Here's how the part is built. I have some questions about the finished solid (model axes, mm). Face numbers are marked on the shaded views. A direction names the side the tool comes from. Give positions to 0.01 mm unless a question says otherwise; leave off trailing zeros. Loops run counter-clockwise (first coordinate to the right, second up) from the corner with the lowest first, then second, coordinate; pieces in that order, holes last. Notation, with made-up numbers: (-8, 89.25) - (27, 89.25) arc R35 ccw to (27, 126.25) - close; hole circle Ø5 at (19, 24). An arc over 180 degrees is marked (long way). Use a Markdown table: item, result.
from build123d import *

# Parameters (mm, degrees)
SKETCH1_W           = 12.5
SKETCH1_H           = 127
BOSS_EXTRUDE1_DEPTH = 106
SKETCH2_W           = 12.5
SKETCH2_H           = 35.5
CUT_EXTRUDE1_DEPTH  = 200
FILLET3_R           = 8
FILLET4_R           = 10
FILLET5_R           = 40
SKETCH5_R           = 3.5
CUT_EXTRUDE5_DEPTH  = 25
CUT_EXTRUDE6_START  = -6
SKETCH5_3_R         = 9.5
SKETCH5_3_R_2       = 3.5
CUT_EXTRUDE6_DEPTH  = 7
SKETCH4_R           = 1.55
CUT_EXTRUDE7_DEPTH  = 16


with BuildPart() as part:
    # Sketch1 → Boss-Extrude1 (new body)
    with BuildSketch(Plane.XY):
        Polygon((0, 8), (0, 0), (228, 0), (228, 8), (178.113248654, 8), (178.113248654, 7), (181, 2), (161, 2), (163.886751346, 7), (163.886751346, 8), (64.113248654, 8), (64.113248654, 7), (67, 2), (47, 2), (49.886751346, 7), (49.886751346, 8), align=None)
        with Locations((234.25, 63.5)):
            Rectangle(SKETCH1_W, SKETCH1_H)
        with Locations((-6.25, 63.5)):
            Rectangle(SKETCH1_W, SKETCH1_H)
    extrude(amount=-BOSS_EXTRUDE1_DEPTH)

    # Sketch2 → Cut-Extrude1 (cut)
    with BuildSketch(Plane(origin=(0, 127, 0), x_dir=(1, 0, 0), z_dir=(0, 1, 0))):
        with Locations((-6.25, 88.25)):
            Rectangle(SKETCH2_W, SKETCH2_H)
        with Locations((-6.25, 17.75)):
            Rectangle(SKETCH2_W, SKETCH2_H)
        with Locations((234.25, 88.25)):
            Rectangle(SKETCH2_W, SKETCH2_H)
        with Locations((234.25, 17.75)):
            Rectangle(SKETCH2_W, SKETCH2_H)
        with BuildLine():
            Line((109.95, 20), (109.95, 86))
            ThreePointArc((109.95, 86), (114, 90.05), (118.05, 86))
            Line((118.05, 86), (118.05, 20))
            ThreePointArc((118.05, 20), (114, 15.95), (109.95, 20))
        make_face()
    extrude(amount=-CUT_EXTRUDE1_DEPTH, mode=Mode.SUBTRACT)

    # Fillet3
    fillet3_edges = [part.edges().sort_by_distance(p)[0] for p in [
        (-6.25, 127, -35.5),
        (234.25, 127, -70.5),
        (234.25, 127, -35.5),
        (-6.25, 127, -70.5),
    ]]
    fillet(fillet3_edges, radius=FILLET3_R)

    # Fillet4
    fillet4_edges = [part.edges().sort_by_distance(p)[0] for p in [
        (228, 8, -53),
        (240.5, 0, -53),
        (0, 8, -53),
        (-12.5, 0, -53),
    ]]
    fillet(fillet4_edges, radius=FILLET4_R)

    # Fillet5
    # the kernel refuses this fillet: 40 mm, written as the material it takes off along each edge
    with BuildSketch(Plane(origin=(228, 107.36517247, -106), x_dir=(-1, 0, 0), z_dir=(0, -1, 0))) as fillet5_piece_1:
        with BuildLine():
            CenterArc((39.746068988, -40), FILLET5_R, 90, 83.540550223)
            Line((0, -35.5), (-0.79492138, -35.41))
            ThreePointArc((-0.79492138, -35.41), (-0.8, -17.75), (-0.8, 0))
            Line((-0.8, 0), (0, 0.8))
            Line((0, 0.8), (39.746068988, 0.8))
            Line((39.746068988, 0.8), (39.746068988, 0))
        make_face()
    extrude(amount=206.73034494, mode=Mode.SUBTRACT)
    with BuildSketch(Plane(origin=(0, 107.36517247, -106), x_dir=(0, 0, 1), z_dir=(0, -1, 0))) as fillet5_piece_2:
        with BuildLine():
            CenterArc((40, -39.746068988), FILLET5_R, 96.459449777, 83.540550223)
            Line((0, -39.746068988), (-0.8, -39.746068988))
            Line((-0.8, -39.746068988), (-0.8, 0))
            Line((-0.8, 0), (0, 0.8))
            ThreePointArc((0, 0.8), (17.75, 0.8), (35.41, 0.79492138))
            Line((35.41, 0.79492138), (35.5, 0))
        make_face()
    extrude(amount=206.73034494, mode=Mode.SUBTRACT)
    with BuildSketch(Plane(origin=(0, 107.36517247, 0), x_dir=(0, 0, -1), z_dir=(0, -1, 0))) as fillet5_piece_3:
        with BuildLine():
            CenterArc((40, 39.746068988), FILLET5_R, 180, 83.540550223)
            Line((0, 39.746068988), (-0.8, 39.746068988))
            Line((-0.8, 39.746068988), (-0.8, 0))
            Line((-0.8, 0), (0, -0.8))
            ThreePointArc((0, -0.8), (17.75, -0.8), (35.41, -0.79492138))
            Line((35.41, -0.79492138), (35.5, 0))
        make_face()
    extrude(amount=206.73034494, mode=Mode.SUBTRACT)
    with BuildSketch(Plane(origin=(228, 107.36517247, 0), x_dir=(-1, 0, 0), z_dir=(0, -1, 0))) as fillet5_piece_4:
        with BuildLine():
            CenterArc((39.746068988, 40), FILLET5_R, 186.459449777, 83.540550223)
            Line((0, 35.5), (-0.79492138, 35.41))
            ThreePointArc((-0.79492138, 35.41), (-0.8, 17.75), (-0.8, 0))
            Line((-0.8, 0), (0, -0.8))
            Line((0, -0.8), (39.746068988, -0.8))
            Line((39.746068988, -0.8), (39.746068988, 0))
        make_face()
    extrude(amount=206.73034494, mode=Mode.SUBTRACT)

    # Sketch5 → Cut-Extrude5 (cut)
    with BuildSketch(Plane(origin=(0, 0, 0), x_dir=(0, 0, -1), z_dir=(1, 0, 0))):
        with Locations((53, 108.5)):
            Circle(SKETCH5_R)
    extrude(amount=-CUT_EXTRUDE5_DEPTH, mode=Mode.SUBTRACT)

    # Sketch5<3> → Cut-Extrude6 (cut)
    with BuildSketch(Plane(origin=(0, 0, 0), x_dir=(0, 0, -1), z_dir=(1, 0, 0)).offset(CUT_EXTRUDE6_START)):
        with Locations((53, 108.5)):
            Circle(SKETCH5_3_R)
        with Locations((53, 108.5)):
            Circle(SKETCH5_3_R_2, mode=Mode.SUBTRACT)
    extrude(amount=-CUT_EXTRUDE6_DEPTH, mode=Mode.SUBTRACT)

    # Sketch4 → Cut-Extrude7 (cut)
    with BuildSketch(Plane(origin=(240.5, 0, 0), x_dir=(0, 0, -1), z_dir=(1, 0, 0))):
        with Locations((40.625, 120.875)):
            Circle(SKETCH4_R)
        with Locations((40.625, 96.125)):
            Circle(SKETCH4_R)
        with Locations((65.375, 96.125)):
            Circle(SKETCH4_R)
        with Locations((65.375, 120.875)):
            Circle(SKETCH4_R)
    extrude(amount=-CUT_EXTRUDE7_DEPTH, mode=Mode.SUBTRACT)


solid = part.part
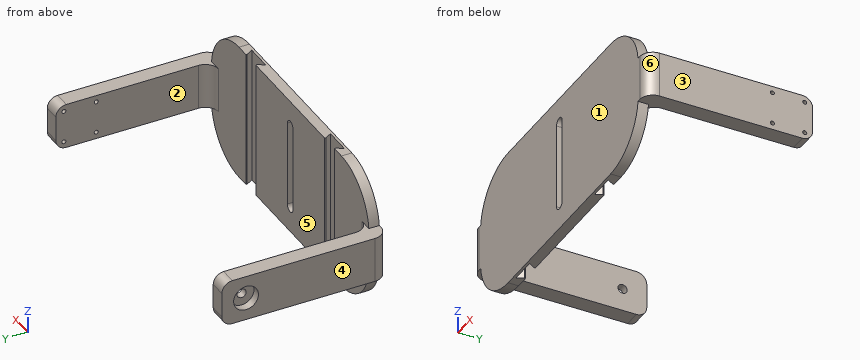
(1) We'd pull the mould along X, two halves only. Please class the marked faces 1, 2, 3 and 4: pulls with the +X half, pulls with the -X half, needs draft (parallel to the pull), parting line crosses it, or undercut.
A:
| item | result |
|---|---|
| face 1 | needs draft |
| face 2 | undercut |
| face 3 | pulls with the +X half |
| face 4 | pulls with the -X half |
(2) Suppose I cut it at B-B on y = 108.5. Write out the boundary of the cut face in (x, z), plus the area to 4 significant figures.
A:
| item | result |
|---|---|
| outline | (-12.5, -70.5) - (0, -70.5) - (0, -56.5) - (-6, -56.5) - (-6, -62.5) - (-12.5, -62.5) - close; (-12.5, -43.5) - (-6, -43.5) - (-6, -49.5) - (0, -49.5) - (0, -35.5) - (-12.5, -35.5) - close; (228, -70.5) - (240.5, -70.5) - (240.5, -35.5) - (228, -35.5) - close |
| area | 709.5 mm2 |
(3) Suppose I cut it at A-A on x = 114. Write out the boundary of the cut face in (y, z).
A:
| item | result |
|---|---|
| outline | (0, -106) - (8, -106) - (8, -90.05) - (0, -90.05) - close; (0, -15.95) - (8, -15.95) - (8, 0) - (0, 0) - close |
(4) Suppose I cut it at C-C on y = 47. Write out the boundary of the cut face in (x, z), plus the area to 3 significant figures.
A:
| item | result |
|---|---|
| outline | (-12.5, -70.5) - (0, -70.5) - (0, -35.5) - (-12.5, -35.5) - close; (228, -70.5) - (240.5, -70.5) - (240.5, -35.5) - (228, -35.5) - close |
| area | 875 mm2 |
(5) Will these pins go through, and if not, where does the flat tip stop? pin 1 (22 mm diameter, centred on x = 52.5, z = -59, fed in from +Y); pin 2 (25 mm diameter, centred on x = 224.5, y = 75.5, fed in from +Z); pin 3 (5.5 mm diameter, centred on y = 108.5, z = -53, fed in from -X).
A:
| item | result |
|---|---|
| pin 1 | y = 8 |
| pin 2 | z = -35.5 |
| pin 3 | x = 228 |
(6) On a 3-axis mill with a long thin cutter (end or side, diameter ignored), from which of +Z, -Z, +X, -X, +Y, -Y can I reach the whole of each face in a straight line? I mean the marked faces 5 and 6. Say none if no direction works.
A:
| item | result |
|---|---|
| face 5 | +Z, -Z, +Y |
| face 6 | +Z, -Z, +X, -Y |
(7) If I drill on line 1 (X direction, y = 111, z = -50); line 2 (X direction, y = 101, z = -46); line 3 (Y direction, x = 141, z = -54.5), over which ranges is the centre line in solid material (lowest first)?
A:
| item | result |
|---|---|
| line 1 | -6 to 0, 228 to 240.5 |
| line 2 | -12.5 to 0, 228 to 240.5 |
| line 3 | 0 to 8 |
